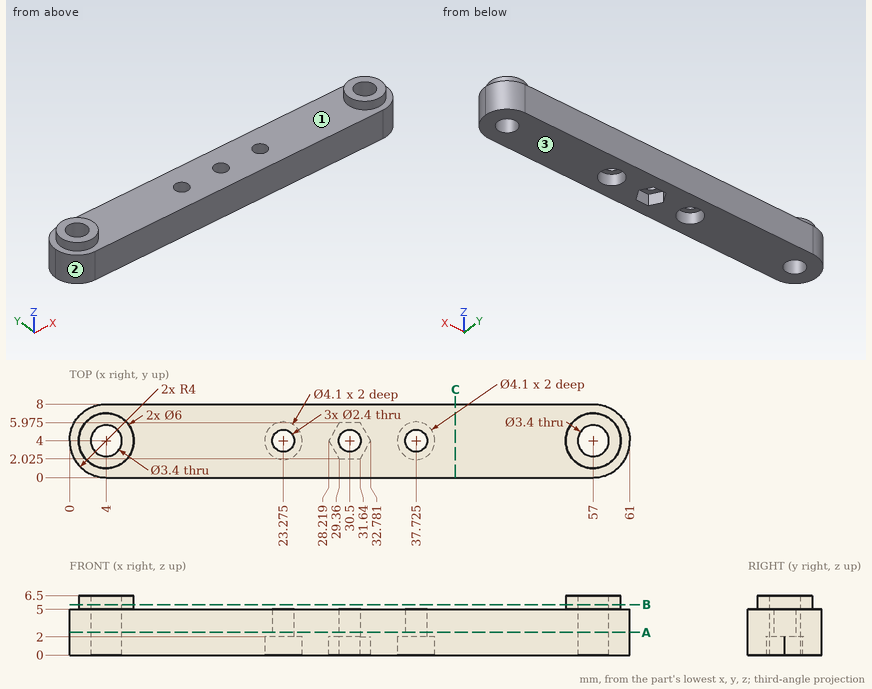
Could you check a few things on this drawing? It's one solid part, dimensions in mm from its lowest x, y, z. Coordinates: 2 decimals unless noted, no trailing zeros. Order: outer loops, then holes, each group sorted by start corner. A loop starts at its lowest first (then second) coordinate and runs counter-clockwise, first axis right, second up. Notation, with made-up numbers: M -31.75,79.25 L 23.25,79.25 A30 ccw 23.25,110.25 Z; hole C 37,-6 d1. An arc over 180 degrees is marked long. Use a Markdown table: item, result. Add a question column.
Q1. I want a section at A-A on z = 2.5. Give the number of separate pieces and of enclosed holes in the cut face.
Q2. I want a section at C-C on x = 42. List the corners of the cut face in (y, z) for me.
Q3. We'd pull the mould along X, two halves only. Please class the marked faces 1, 2 and 3: pulls with the +X half, pulls with the -X half, needs draft (parallel to the pull), parting line crosses it, or undercut.
Q4. If I drill on L1, parallel to X at y = 4.75, z = 3.25 (1 decimal); L2, parallel to Y at x = 4, z = 2.75; L3, parallel to Z at x = 38, y = 5.25, over which ranges is the centre line in solid material (lowest first)?
Q5. I'm going to push flat-ended pins straight in: pin 1 (2.5 mm diameter, centred on x = 41, y = 4.5, fed in from +Z); pin 2 (3 mm diameter, centred on x = 30.5, y = 4, fed in from -Z); pin 3 (2 mm diameter, centred on y = 2.5, z = 2, fed in from -X). Where does each tip first touch, or does it pass through?
Q6. I want a section at B-B on z = 5.5. List the corners of the cut face in (x, y) for me.
Checked values:
| question | item | result |
|---|---|---|
| 1 | separate pieces | 1 |
| 1 | enclosed holes | 5 |
| 2 | outline | M 0,0 L 8,0 L 8,5 L 0,5 Z |
| 3 | face 1 | undercut |
| 3 | face 2 | pulls with the -X half |
| 3 | face 3 | needs draft |
| 4 | L1 | 0.1 to 2.5, 5.5 to 22.3, 24.2 to 29.6, 31.4 to 36.8, 38.7 to 55.5, 58.5 to 60.9 |
| 4 | L2 | 0 to 2.3, 5.7 to 8 |
| 4 | L3 | 2 to 5 |
| 5 | pin 1 | z = 5 |
| 5 | pin 2 | z = 2 |
| 5 | pin 3 | x = 0.03 |
| 6 | outline | C 4,4 d6; C 57,4 d6; hole C 4,4 d3.4; hole C 57,4 d3.4 |
